Design review of the part built by this model. Coordinates are the model's own, in mm. Round coordinates to 2 decimals unless told otherwise and drop trailing zeros. Answer as CSV lines item,"result". Start each with the question number.
```python
from build123d import *

# Parameters (mm, degrees)
F0_W     = 65
F0_H     = 65
F1_DEPTH = 7
F2_W     = 65
F2_H     = 65
F3_DEPTH = 5
F4_R     = 2.1
F5_DEPTH = 39


with BuildPart() as f1:
    # F0 (on Top) → F1 (new body)
    with BuildSketch(Plane.XY):
        Rectangle(F0_W, F0_H)
    extrude(amount=F1_DEPTH)

    # F2 (on face) → F3 (join)
    with BuildSketch(Plane(origin=(0, 0, 0), x_dir=(1, 0, 0), z_dir=(0, 0, -1))):
        Rectangle(F2_W, F2_H)
    extrude(amount=F3_DEPTH)

    # F4 (on face) → F5 (cut)
    with BuildSketch(Plane.XY.offset(7)):
        with Locations((-28.980361, 29.262956)):
            Circle(F4_R)
        with Locations((29.019639, 29.262956)):
            Circle(F4_R)
        with Locations((29.019639, -28.737044)):
            Circle(F4_R)
        with Locations((-28.980361, -28.737044)):
            Circle(F4_R)
    extrude(amount=-F5_DEPTH, mode=Mode.SUBTRACT)


solid = f1.part
```
Q1. Mouldability with a two-part tool opening along X and no side actions: class faces 1 (the cylindrical face through (-31.08, 29.36, 1.08)), 2 (the flat face through (32.5, 0, 1)), 3 (the flat face through (0, 32.5, 1)) as pulls with the +X half, pulls with the -X half, needs draft (parallel to the pull), parting line crosses it, or undercut.
Q2. To check wall thickness, follow probe 1 along X at (y, z) = (30, 0.25). State the ranges of the line that lie inside material, in increasing order. Write a range as from..to.
Q3. For pin 1 Ø6.5 at (x, y) = (-28.98, 29.26) entering from +Z; pin 2 Ø3.5 at (x, y) = (-28.98, -28.74) entering from +Z, all flat-tipped, find the tip position at first contact; note any pin that passes through.
Worked answers:
1,face 1,"undercut"
1,face 2,"pulls with the +X half"
1,face 3,"needs draft"
2,probe 1,"x = -32.5..-30.95, -27.01..27.05, 30.99..32.5"
3,pin 1,"stops at z = 7"
3,pin 2,"passes through"
